Part print with two shaded views. Sizes in mm from the minimum x, y, z corner. A direction names the side the tool comes from. Round coordinates to 2 decimals unless told otherwise and drop trailing zeros. Loops run counter-clockwise (first coordinate to the right, second up) from the corner with the lowest first, then second, coordinate; pieces in that order, holes last. Notation, with made-up numbers: (-29, 19.25) - (22, 19.25) arc R36 cw to (22, 53.25) - close; hole circle Ø5 at (48.5, 1). An arc over 180 degrees is marked (long way). Use a Markdown table: item, result.
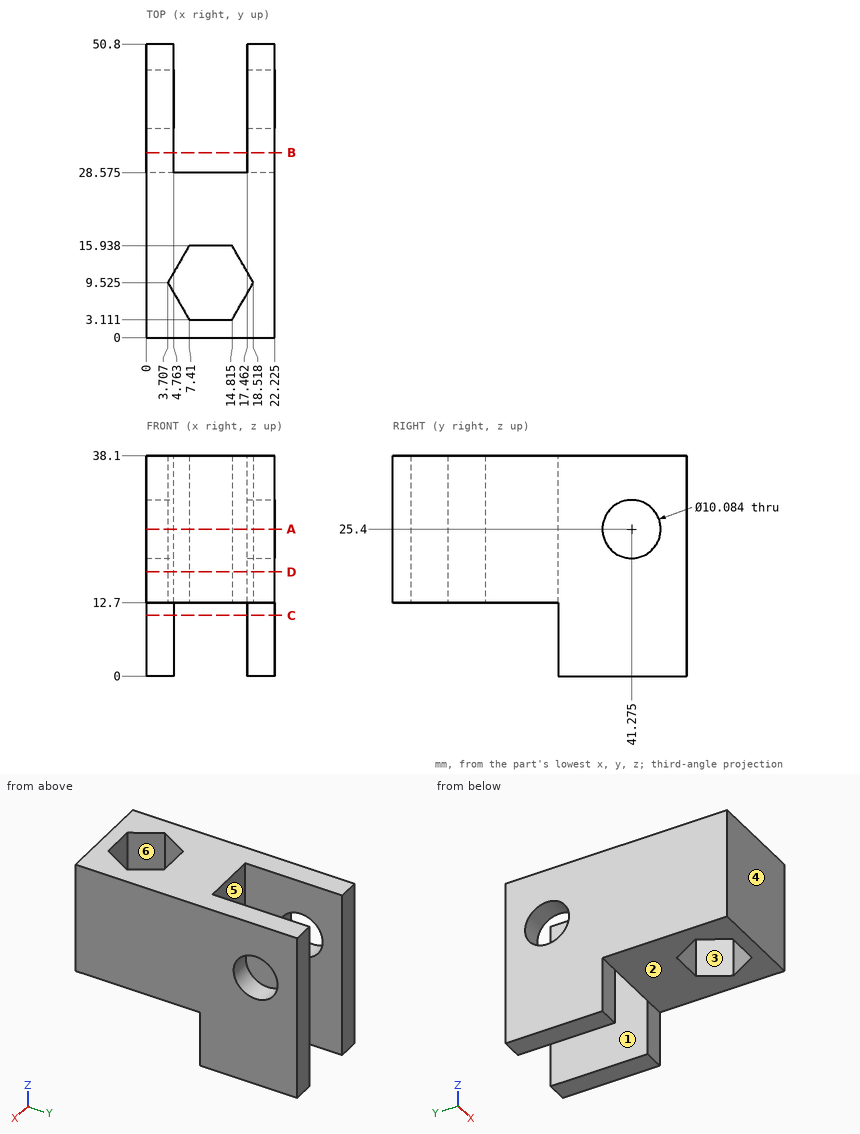
Q1. Cut at C-C, the plane z = 10.5. List the corners of the cut face in (x, y) (1 decimal).
Results found:
| item | result |
|---|---|
| outline | (0, 28.6) - (4.8, 28.6) - (4.8, 50.8) - (0, 50.8) - close; (17.5, 28.6) - (22.2, 28.6) - (22.2, 50.8) - (17.5, 50.8) - close |
Q2. Pull direction Y, two halves, no side cores. Call the marked faces 4, 5 and 6: pulls with the +Y half, pulls with the -Y half, needs draft (parallel to the pull), parting line crosses it, or undercut.
Results found:
| item | result |
|---|---|
| face 4 | pulls with the -Y half |
| face 5 | pulls with the +Y half |
| face 6 | undercut |
Q3. Cut at A-A, the plane z = 25.4. List the corners of the cut face in (x, y) (1 decimal), plus the area to 3 significant figures.
Results found:
| item | result |
|---|---|
| outline | (0, 0) - (22.2, 0) - (22.2, 36.2) - (17.5, 36.2) - (17.5, 28.6) - (4.8, 28.6) - (4.8, 36.2) - (0, 36.2) - close; (0, 46.3) - (4.8, 46.3) - (4.8, 50.8) - (0, 50.8) - close; (17.5, 46.3) - (22.2, 46.3) - (22.2, 50.8) - (17.5, 50.8) - close; hole (3.7, 9.5) - (7.4, 3.1) - (14.8, 3.1) - (18.5, 9.5) - (14.8, 15.9) - (7.4, 15.9) - close |
| area | 608 mm2 |
Q4. Cut at D-D, the plane z = 18. List the corners of the cut face in (x, y) (1 decimal).
Results found:
| item | result |
|---|---|
| outline | (0, 0) - (22.2, 0) - (22.2, 50.8) - (17.5, 50.8) - (17.5, 28.6) - (4.8, 28.6) - (4.8, 50.8) - (0, 50.8) - close; hole (3.7, 9.5) - (7.4, 3.1) - (14.8, 3.1) - (18.5, 9.5) - (14.8, 15.9) - (7.4, 15.9) - close |
Q5. Drop flat-ended pins along their axis: pin 1 (11.5 mm diameter, centred on y = 41.275, z = 25.4, fed in from -X); pin 2 (4 mm diameter, centred on x = 20, z = 6, fed in from -Y) (1 decimal); pin 3 (11 mm diameter, centred on x = 11, y = 13, fed in from -Z); pin 4 (2 mm diameter, centred on x = 11, z = 30, fed in from +Y) (1 decimal). Give the stop position or say it passes through.
Results found:
| item | result |
|---|---|
| pin 1 | stops at x = 0 |
| pin 2 | stops at y = 28.6 |
| pin 3 | stops at z = 12.7 |
| pin 4 | stops at y = 28.6 |
Q6. Which spindle directions (+Z, -Z, +X, -X, +Y, -Y) get a long thin tool onto all of the face, cutting with end or side? Do the marked faces 1, 2 and 3. Say none if no direction does.
Results found:
| item | result |
|---|---|
| face 1 | +Z, -Z, +Y |
| face 2 | -Z, +X, -X, -Y |
| face 3 | +Z, -Z |
Q7. Probe line 1 (X direction, y = 41.5, z = 10.5) (1 decimal); line 2 (Y direction, x = 1.45, z = 25.4); line 3 (Y direction, x = 9.75, z = 25) (1 decimal). List the from-to ranges inside material, lowest first.
Results found:
| item | result |
|---|---|
| line 1 | x = 0 to 4.8, 17.5 to 22.2 |
| line 2 | y = 0 to 36.23, 46.32 to 50.8 |
| line 3 | y = 0 to 3.1, 15.9 to 28.6 |
Q8. Cut at B-B, the plane y = 32. List the corners of the cut face in (x, z) (1 decimal).
Results found:
| item | result |
|---|---|
| outline | (0, 0) - (4.8, 0) - (4.8, 38.1) - (0, 38.1) - close; (17.5, 0) - (22.2, 0) - (22.2, 38.1) - (17.5, 38.1) - close |
